Autodesk Inventor part; units mm, degrees
ref_plane "YZ Plane" through (0, 0, 0) normal (1, 0, 0) x (0, 1, 0)
ref_plane "XZ Plane" through (0, 0, 0) normal (0, 1, 0) x (-1, 0, 0)
ref_plane "XY Plane" through (0, 0, 0) normal (0, 0, 1) x (1, 0, 0)
sketch "スケッチ1" plane through (0, 0, 0) normal (1, 0, 0) x (0, 1, 0)
  point P0 (0, 0)
sketch "スケッチ2" plane through (0, 0, 0) normal (1, 0, 0) x (0, 1, 0)
  circle A0 centre (0, 0) radius 28.4
  dimension "d0" = 56.8
extrude "押し出し1" add sketch "スケッチ2" along normal blind 6
sketch "スケッチ3" plane through (6, 0, 0) normal (1, 0, 0) x (0, 0, -1)
  circle A0 centre (0, 0) radius 12
  dimension "d3" = 24
extrude "押し出し2" add sketch "スケッチ3" along normal blind 20.4
sketch "スケッチ8" plane through (26.4, 0, 0) normal (1, 0, 0) x (0, 0, -1)
  circle A0 centre (0, 0) radius 12
hole "穴2" at (26.4, 0, 0) direction (-1, 0, 0) diameter 6 end through all
sketch "スケッチ7" plane through (0, 0, 0) normal (-1, 0, 0) x (0, 0, 1)
  circle A0 centre (0, 0) radius 23.75
  line L0 (0, -23.75) -> (-20.5681, -11.875)
  line L1 (-20.5681, -11.875) -> (-20.5681, 11.875)
  line L2 (-20.5681, 11.875) -> (0, 23.75)
  line L3 (0, 23.75) -> (20.5681, 11.875)
  line L4 (20.5681, 11.875) -> (20.5681, -11.875)
  line L5 (20.5681, -11.875) -> (0, -23.75)
  dimension "d43" = 47.5
hole "穴3" at (0, 11.875, 20.5681) at (0, 23.75, 0) at (0, -11.875, 20.5681) at (0, -23.75, 0) at (0, -11.875, -20.5681) at (0, 11.875, -20.5681) direction (1, 0, 0) diameter 5.2 end through all
properties part number "10mmkethub18025"
Verification items for the finished model (mm, model axes). A direction names the side the tool comes from. Round coordinates to 2 decimals unless told otherwise and drop trailing zeros. Loops run counter-clockwise (first coordinate to the right, second up) from the corner with the lowest first, then second, coordinate; pieces in that order, holes last. Notation, with made-up numbers: (-1.5, 17) - (30.5, 17) arc R17 cw to (30.5, 23) - close; hole circle Ø9 at (11.5, 76). An arc over 180 degrees is marked (long way). Use one line per item in the form item = value.
1. Section check A-A on z = 0. Record the cut outline in (x, y), and give its area (3 significant figures).
A:
outline = (0, -28.4) - (6, -28.4) - (6, -26.35) - (0, -26.35) - close; (0, -21.15) - (6, -21.15) - (6, -12) - (26.4, -12) - (26.4, -3) - (0, -3) - close; (0, 3) - (26.4, 3) - (26.4, 12) - (6, 12) - (6, 21.15) - (0, 21.15) - close; (0, 26.35) - (6, 26.35) - (6, 28.4) - (0, 28.4) - close
area = 610 mm²
2. Draft check along Y on faces 3 (the flat face through (26.4, -2.5, -2.5)), 4 (the cylindrical face through (3.04, -9.57, 21.77)), 5 (the cylindrical face through (16.06, -0.53, 11.99)), 6 (the cylindrical face through (3.04, 14.18, 21.77)). Enter one of: pulls with the +Y half, pulls with the -Y half, needs draft (parallel to the pull), parting line crosses it, or undercut.
A:
face_3 = needs draft
face_4 = undercut
face_5 = parting line crosses it
face_6 = undercut
3. Section check B-B on y = -13. Record the cut outline in (x, z).
A:
outline = (0, -25.25) - (6, -25.25) - (6, -22.91) - (0, -22.91) - close; (0, -18.22) - (6, -18.22) - (6, 18.22) - (0, 18.22) - close; (0, 22.91) - (6, 22.91) - (6, 25.25) - (0, 25.25) - close
4. Section check C-C on y = -23.75. Record the cut outline in (x, z).
A:
outline = (0, -15.57) - (6, -15.57) - (6, -2.6) - (0, -2.6) - close; (0, 2.6) - (6, 2.6) - (6, 15.57) - (0, 15.57) - close
5. Section check D-D on x = 19.25. Record the cut outline in (y, z).
A:
outline = circle Ø24 at (0, 0); hole circle Ø6 at (0, 0)
6. Scan lines: probe 1 along X at (y, z) = (-2.5, 23.5); probe 2 along Y at (x, z) = (21.5, 0.5); probe 3 along Z at (x, y) = (4.2, 23.75). Record each from-to range of solid material in increasing order.
A:
probe_1 = 0 to 6
probe_2 = -11.99 to -2.96, 2.96 to 11.99
probe_3 = -15.57 to -2.6, 2.6 to 15.57
7. Access from +Z, -Z, +X, -X, +Y, -Y to the whole of each face (thin tool, end or side, straight path). Record for faces 1 (the cylindrical face through (2.958, -3.697, -28.158)), 2 (the flat face through (6, -0.4, -12.2)).
A:
face_1 = +X, -X
face_2 = +X
8. Gauge pin test, flat ends, axial feed: pin 1 Ø3 at (x, z) = (5.5, -21.5) entering from +Y; pin 2 Ø6 at (y, z) = (11.88, -20.57) entering from +X; pin 3 Ø12 at (x, y) = (22, -8.5) entering from +Z. Record the tip position at first contact, or that the pin passes through.
A:
pin_1 = 20.16
pin_2 = 6
pin_3 = 11.74
